Read the model definition and answer for the solid it produces. Units are mm, in the model's axes. A direction names the side the tool comes from. Coordinates: 2 decimals unless noted, no trailing zeros. Order: outer loops, then holes, each group sorted by start corner. A loop starts at its lowest first (then second) coordinate and runs counter-clockwise, first axis right, second up.
```python
from build123d import *

# Parameters (mm, degrees)
SKETCH1_R               = 34.5
SKETCH1_R_2             = 4
BOSS_EXTRUDE1_DEPTH     = 4.5
SKETCH2_W               = 1.5
SKETCH2_H               = 2.65
CUT_EXTRUDE1_DEPTH      = 49.997448913
CUT_EXTRUDE1_DEPTH_BACK = 49.997448913
SKETCH4_W               = 1.55
SKETCH4_H               = 1.5
SKETCH5_W               = 1.5
SKETCH5_H               = 1.55
CUT_EXTRUDE2_DEPTH      = 49.997448913


with BuildPart() as part:
    # Sketch1 → Boss-Extrude1 (new body)
    with BuildSketch(Plane.XY):
        Circle(SKETCH1_R)
        with Locations((5.75, 5.75)):
            Circle(SKETCH1_R_2, mode=Mode.SUBTRACT)
        with Locations((8.338190451, 15.409258263)):
            Circle(SKETCH1_R_2, mode=Mode.SUBTRACT)
        with Locations((17.997448714, 17.997448714)):
            Circle(SKETCH1_R_2, mode=Mode.SUBTRACT)
        with Locations((15.409258263, 8.338190451)):
            Circle(SKETCH1_R_2, mode=Mode.SUBTRACT)
        with Locations((25.068516526, 5.75)):
            Circle(SKETCH1_R_2, mode=Mode.SUBTRACT)
        with Locations((5.75, 25.068516526)):
            Circle(SKETCH1_R_2, mode=Mode.SUBTRACT)
        with Locations((25.068556101, -5.749960425)):
            Circle(SKETCH1_R_2, mode=Mode.SUBTRACT)
        with Locations((15.409297838, -8.338150876)):
            Circle(SKETCH1_R_2, mode=Mode.SUBTRACT)
        with Locations((17.997488289, -17.997409139)):
            Circle(SKETCH1_R_2, mode=Mode.SUBTRACT)
        with Locations((8.338230026, -15.409218688)):
            Circle(SKETCH1_R_2, mode=Mode.SUBTRACT)
        with Locations((5.750039575, -25.068476951)):
            Circle(SKETCH1_R_2, mode=Mode.SUBTRACT)
        with Locations((5.750039575, -5.749960425)):
            Circle(SKETCH1_R_2, mode=Mode.SUBTRACT)
        with Locations((-5.74992085, -25.068516526)):
            Circle(SKETCH1_R_2, mode=Mode.SUBTRACT)
        with Locations((-8.338111301, -15.409258263)):
            Circle(SKETCH1_R_2, mode=Mode.SUBTRACT)
        with Locations((-17.997369564, -17.997448714)):
            Circle(SKETCH1_R_2, mode=Mode.SUBTRACT)
        with Locations((-15.409179113, -8.338190451)):
            Circle(SKETCH1_R_2, mode=Mode.SUBTRACT)
        with Locations((-25.068437376, -5.75)):
            Circle(SKETCH1_R_2, mode=Mode.SUBTRACT)
        with Locations((-5.74992085, -5.75)):
            Circle(SKETCH1_R_2, mode=Mode.SUBTRACT)
        with Locations((-25.068476951, 5.749960425)):
            Circle(SKETCH1_R_2, mode=Mode.SUBTRACT)
        with Locations((-15.409218688, 8.338150876)):
            Circle(SKETCH1_R_2, mode=Mode.SUBTRACT)
        with Locations((-17.997409139, 17.997409139)):
            Circle(SKETCH1_R_2, mode=Mode.SUBTRACT)
        with Locations((-8.338150876, 15.409218688)):
            Circle(SKETCH1_R_2, mode=Mode.SUBTRACT)
        with Locations((-5.749960425, 25.068476951)):
            Circle(SKETCH1_R_2, mode=Mode.SUBTRACT)
        with Locations((-5.749960425, 5.749960425)):
            Circle(SKETCH1_R_2, mode=Mode.SUBTRACT)
    extrude(amount=BOSS_EXTRUDE1_DEPTH)

    # Sketch2 → Cut-Revolve1 (revolve, cut)
    with BuildSketch(Plane(origin=(0, 0, 0), x_dir=(0, 0, -1), z_dir=(1, 0, 0))):
        with Locations((-0.75, 33.175)):
            Rectangle(SKETCH2_W, SKETCH2_H)
        with Locations((-3.75, 33.175)):
            Rectangle(SKETCH2_W, SKETCH2_H)
    revolve(axis=Axis((0, 0, 0), (0, 0, 1)), mode=Mode.SUBTRACT)

    # Sketch4 → Cut-Extrude1 (cut, two sides: drawn at the far end of the back side and taken through both)
    with BuildSketch(Plane(origin=(0, 0, 0), x_dir=(1, 0, 0), z_dir=(0, 1, 0)).offset(-CUT_EXTRUDE1_DEPTH_BACK)):
        with Locations((0, -0.75)):
            Rectangle(SKETCH4_W, SKETCH4_H)
    extrude(amount=CUT_EXTRUDE1_DEPTH + CUT_EXTRUDE1_DEPTH_BACK, mode=Mode.SUBTRACT)

    # Sketch5 → Cut-Extrude2 (cut, through all)
    with BuildSketch(Plane(origin=(0, 0, 0), x_dir=(0, 0, -1), z_dir=(1, 0, 0))):
        with Locations((-0.75, 0)):
            Rectangle(SKETCH5_W, SKETCH5_H)
    extrude(amount=-CUT_EXTRUDE2_DEPTH, mode=Mode.SUBTRACT)


solid = part.part
```
1) A cutting plane is placed at B-B, the plane y = -3. State how many separate pieces and enclosed holes the cut face has, and give its area (3 significant figures).
A:
separate pieces: 5
enclosed holes: 0
area: 186 mm2
2) A cutting plane is placed at D-D, the plane x = -26.5. Determine the outline of the cut face in (y, z) (3 decimals), and give its area (3 significant figures).
A:
outline: (-22.091, 1.5) - (-17.668, 1.5) - (-17.668, 0) - (-9.485, 0) - (-9.485, 4.5) - (-17.668, 4.5) - (-17.668, 3) - (-22.091, 3) - close; (-2.015, 0) - (-0.775, 0) - (-0.775, 1.5) - (0.775, 1.5) - (0.775, 0) - (2.015, 0) - (2.015, 4.5) - (-2.015, 4.5) - close; (9.485, 0) - (17.668, 0) - (17.668, 1.5) - (22.091, 1.5) - (22.091, 3) - (17.668, 3) - (17.668, 4.5) - (9.485, 4.5) - close
area: 103 mm2
3) Flat-ended cylindrical pins translate along their axes: pin 1 Ø6.5 at (x, y) = (5.75, 5.75) entering from +Z; pin 2 Ø0.8 at (y, z) = (13, 1) entering from +X; pin 3 Ø1.5 at (x, z) = (-4, 1.5) entering from +Y; pin 4 Ø0.8 at (y, z) = (-3.5, 0.5) entering from -X. Find the tip coordinate at first contact, or state that the pin passes through.
A:
pin 1: passes through
pin 2: stops at x = 29.25
pin 3: stops at y = 34.35
pin 4: stops at x = -31.7
4) Determine the mould class of faces 1 (the flat face through (-13, -16, 0)), 2 (the cylindrical face through (5.16, 12.98, 2.22)), 3 (the cylindrical face through (32.907, 10.363, 2.24)) for opening direction Y: pulls with the +Y half, pulls with the -Y half, needs draft (parallel to the pull), parting line crosses it, or undercut.
A:
face 1: needs draft
face 2: undercut
face 3: parting line crosses it
5) Which of the six approach directions +Z, -Z, +X, -X, +Y, -Y give full straight-line access (tool end or side, diameter ignored) to faces 4 (the cylindrical face through (31.843, -0.69, 0.74)), 5 (the flat face through (-3, 0, 1.5)), 6 (the cylindrical face through (19.225, -7.137, 2.218)), 7 (the flat face through (0.775, 0, 1))?
A:
face 4: -Z, +X
face 5: -Z
face 6: +Z, -Z
face 7: -Z, +Y, -Y
6) Straight lines are drawn through the part: line 1 (X direction, y = 4, z = 0.2) (3 decimals); line 2 (Y direction, x = -28.5, z = 3.85); line 3 (Y direction, x = 18, z = 4.25). For each, find the intervals that lie inside material, in ascending order.
A:
line 1: x = -31.598 to -28.665, -21.472 to -9.347, -2.153 to -0.775, 0.775 to 2.153, 9.347 to 21.472, 28.665 to 31.598
line 2: y = -14.22 to -7.81, -3.69 to 3.69, 7.81 to 14.22
line 3: y = -26.28 to -22, -14 to -11.39, -5.29 to 5.29, 11.39 to 14, 22 to 26.28
7) A cutting plane is placed at A-A, the plane x = 3.5. Determine the outline of the cut face in (y, z), and give its area (3 significant figures).
A:
outline: (-34.32, 1.5) - (-31.66, 1.5) - (-31.66, 0) - (-28.38, 0) - (-28.38, 4.5) - (-31.66, 4.5) - (-31.66, 3) - (-34.32, 3) - close; (-21.76, 0) - (-9.06, 0) - (-9.06, 4.5) - (-21.76, 4.5) - close; (-2.44, 0) - (2.44, 0) - (2.44, 4.5) - (-2.44, 4.5) - close; (9.06, 0) - (21.76, 0) - (21.76, 4.5) - (9.06, 4.5) - close; (28.38, 0) - (31.66, 0) - (31.66, 1.5) - (34.32, 1.5) - (34.32, 3) - (31.66, 3) - (31.66, 4.5) - (28.38, 4.5) - close
area: 174 mm2
